Autodesk Inventor part; units mm, degrees
ref_plane "Work Plane1" through (144.7964, 60.3681, 0) normal (0.9790451, 0.2036437, 0) x (-0.2036437, 0.9790451, 0)
ref_plane "YZ Plane" through (0, 0, 0) normal (1, 0, 0) x (0, 1, 0)
ref_plane "XZ Plane" through (0, 0, 0) normal (0, 1, 0) x (-1, 0, 0)
sketch "Main Outline" plane through (0, 0, 0) normal (0, 0, 1) x (1, 0, 0)
  line L0 (0, 0) -> (304.8, 0) construction
  line L1 (304.8, 0) -> (304.8, 50.8) construction
  line L2 (304.8, 50.8) -> (0, 50.8) construction
  line L3 (0, 50.8) -> (0, 0) construction
  line L4 (0, 50.8) -> (0, 53.34) construction
  line L5 (0, 53.34) -> (304.8, 53.34) construction
  line L6 (304.8, 53.34) -> (304.8, 50.8) construction
  circle A0 centre (152.4, 23.8125) radius 17.4625 construction
  line L7 (152.4, 23.8125) -> (152.4, 0) construction
  circle A1 centre (152.4, 23.8125) radius 27.94 construction
  circle A2 centre (152.4, 23.8125) radius 21.59 construction
  line L8 (152.4, 23.8125) -> (144.7964, 60.3681) construction
  circle A3 centre (144.7964, 60.3681) radius 15.24 construction
  circle A4 centre (144.7964, 60.3681) radius 8.89 construction
  circle A5 centre (144.7964, 60.3681) radius 14.2875 construction
  arc A6 (164.6591, 71.8014) -> (129.0153, 43.7486) centre (144.7964, 60.3681) ccw construction
  circle A7 centre (98.8106, 85.598) radius 32.258 construction
  circle A8 centre (126.6733, 147.4971) radius 32.258 construction
  circle A9 centre (176.9075, 101.8424) radius 32.258 construction
  circle A10 centre (144.7964, 60.3681) radius 11.1125 construction
  circle A11 centre (152.4, 23.8125) radius 49.53 construction
  line L9 (144.7964, 60.3681) -> (126.6733, 147.4971) construction
  line L10 (144.7964, 60.3681) -> (98.8106, 85.598) construction
  line L11 (98.8106, 85.598) -> (176.9075, 101.8424) construction
  line L12 (176.9075, 101.8424) -> (144.7964, 60.3681) construction
  circle A12 centre (98.8106, 85.598) radius 9.5493 construction
  arc A13 (174.9629, 111.1915) -> (185.6989, 98.1139) centre (176.9075, 101.8424) ccw construction
  circle A14 centre (126.6733, 147.4971) radius 9.5493 construction
  line L13 (96.8659, 94.9472) -> (174.9629, 111.1915) construction
  line L14 (185.6989, 98.1139) -> (165.8956, 51.4198) construction
  line L15 (92.2351, 78.6732) -> (129.0153, 43.7486) construction
  line L16 (174.9629, 111.1915) -> (176.9075, 101.8424) construction
  line L17 (176.9075, 101.8424) -> (185.6989, 98.1139) construction
  arc A15 (185.6989, 98.1139) -> (174.9629, 111.1915) centre (176.9075, 101.8424) ccw construction
  arc A16 (165.8956, 51.4198) -> (164.6591, 71.8014) centre (144.7964, 60.3681) ccw construction
  arc A17 (129.0153, 43.7486) -> (165.8956, 51.4198) centre (144.7964, 60.3681) ccw construction
  circle A18 centre (126.6086, 147.808) radius 32.258 construction
  circle A19 centre (126.544, 148.1188) radius 32.258 construction
  circle A20 centre (126.4793, 148.4297) radius 32.258 construction
  line L18 (126.6733, 147.4971) -> (126.4793, 148.4297) construction
  circle A21 centre (126.738, 147.1863) radius 32.258 construction
  circle A22 centre (117.4622, 43.2997) radius 9.525 construction
  circle A23 centre (176.6694, 55.615) radius 9.525 construction
  line L19 (152.4, 23.8125) -> (117.4622, 43.2997) construction
  line L20 (152.4, 23.8125) -> (176.6694, 55.615) construction
  line L21 (117.4622, 43.2997) -> (98.8106, 85.598) construction
  line L22 (176.6694, 55.615) -> (176.9075, 101.8424) construction
  circle A24 centre (135.1821, 106.5897) radius 7.9375 construction
  line L23 (135.6243, 150.8242) -> (166.2787, 68.353) construction
  circle A25 centre (152.4, 23.8125) radius 29.845 construction
  line L24 (117.1381, 146.979) -> (121.9118, 59.1246) construction
  circle A26 centre (99.0889, 85.4453) radius 32.258 construction
  circle A27 centre (97.9755, 86.0562) radius 32.258 construction
  line L25 (97.9755, 86.0562) -> (98.8106, 85.598) construction
  circle A28 centre (98.2538, 85.9034) radius 32.258 construction
  circle A29 centre (98.5322, 85.7507) radius 32.258 construction
  circle A30 centre (152.4, 23.8125) radius 29.845 construction
  circle A31 centre (122.555, 23.8125) radius 6.35 construction
  circle A32 centre (179.7696, 35.7133) radius 6.35 construction
  line L26 (122.555, 23.8125) -> (152.4, 23.8125) construction
  line L27 (152.4, 23.8125) -> (182.245, 23.8125) construction
  circle A33 centre (182.245, 23.8125) radius 6.35 construction
  circle A34 centre (125.0304, 11.9117) radius 6.35 construction
  circle A35 centre (150.4199, 33.3321) radius 39.5684 construction
  line L28 (72.9795, 65.6655) -> (119.7593, 8.3204) construction
  circle A36 centre (177.4906, 102.5955) radius 32.258 construction
  line L29 (176.9075, 101.8424) -> (177.4906, 102.5955) construction
  circle A37 centre (177.2963, 102.3445) radius 32.258 construction
  circle A38 centre (177.1019, 102.0934) radius 32.258 construction
  circle A39 centre (176.7131, 101.5913) radius 32.258 construction
  line L30 (188.5109, 22.6209) -> (208.5442, 93.8632) construction
  circle A40 centre (135.1821, 106.5897) radius 9.5727 construction
  arc A41 (86.8202, 116.3239) -> (96.3065, 136.4856) centre (81.3304, 131.2195) ccw construction
  arc A42 (158.9123, 149.5077) -> (175.6513, 134.801) centre (174.7462, 150.6502) ccw construction
  line L31 (126.4793, 148.4297) -> (126.9966, 145.9429) construction
  line L32 (116.5322, 146.3607) -> (117.0495, 143.8739) construction
  line L33 (136.9437, 148.0119) -> (136.4264, 150.4987) construction
  arc A43 (136.4264, 150.4987) -> (116.5322, 146.3607) centre (126.4793, 148.4297) ccw construction
  arc A44 (117.0495, 143.8739) -> (136.9437, 148.0119) centre (126.9966, 145.9429) ccw construction
  line L34 (177.4906, 102.5955) -> (175.9357, 100.5871) construction
  line L35 (169.4571, 108.8154) -> (167.9021, 106.807) construction
  line L36 (183.9692, 94.3672) -> (185.5242, 96.3756) construction
  arc A45 (185.5242, 96.3756) -> (169.4571, 108.8154) centre (177.4906, 102.5955) ccw construction
  arc A46 (167.9021, 106.807) -> (183.9692, 94.3672) centre (175.9357, 100.5871) ccw construction
  line L37 (97.9755, 86.0562) -> (100.2023, 84.8344) construction
  line L38 (93.0884, 77.1487) -> (95.3153, 75.927) construction
  line L39 (105.0894, 93.7418) -> (102.8625, 94.9636) construction
  arc A47 (102.8625, 94.9636) -> (93.0884, 77.1487) centre (97.9755, 86.0562) ccw construction
  arc A48 (95.3153, 75.927) -> (105.0894, 93.7418) centre (100.2023, 84.8344) ccw construction
  circle A49 centre (117.4622, 43.2997) radius 3.9687 construction
  circle A50 centre (176.6694, 55.615) radius 3.9687 construction
  line L40 (152.4, 23.8125) -> (158.4777, -5.4071) construction
  arc A51 (80.1751, 59.3139) -> (79.0947, 58.1692) centre (79.7097, 58.6709) ccw construction
  arc A52 (205.9254, 84.5503) -> (204.4781, 85.1692) centre (205.1613, 84.7652) ccw construction
  circle A53 centre (152.4, 23.8125) radius 14.224 construction
  circle A54 centre (135.1821, 106.5897) radius 3.9687 construction
  circle A55 centre (156.538, 3.9183) radius 6.35 construction
  circle A56 centre (156.538, 3.9183) radius 2.0828 construction
  circle A57 centre (152.4, 23.8125) radius 20.32 construction
  line L41 (133.1021, 30.1759) -> (152.4, 23.8125) construction
  line L42 (152.4, 23.8125) -> (167.5599, 37.3432) construction
  circle A58 centre (167.5599, 37.3432) radius 2.0828 construction
  circle A59 centre (167.5599, 37.3432) radius 3.9687 construction
  circle A60 centre (133.1021, 30.1759) radius 2.0828 construction
  circle A61 centre (133.1021, 30.1759) radius 3.9688 construction
  point P0 (126.738, 147.1863)
  point P1 (176.7131, 101.5913)
  dimension "d18" = 99.06
  dimension "d58" = 64.516
  dimension "d86" = 64.516
  dimension "d0" = 304.8
  dimension "d1" = 50.8
  dimension "d2" = 2.54
  dimension "d3" = 34.925
  dimension "d4" = 23.8125
  dimension "d5" = 152.4
  dimension "d6" = 55.88
  dimension "d7" = 43.18
  dimension "d8" = 37.338
  dimension "d10" = 30.48
  dimension "d11" = 17.78
  dimension "d12" = 28.575
  dimension "d13" = 45.8366
  dimension "d14" = 64.516
  dimension "d15" = 64.516
  dimension "d16" = 64.516
  dimension "d17" = 22.225
  dimension "d19" = 52.4523
  dimension "d20" = 88.9939
  dimension "d21" = 19.0986
  dimension "d22" = 19.0986
  dimension "d23" = 19.0986
  dimension "d30" = 124.732
  dimension "d40" = 64.516
  dimension "d41" = 64.516
  dimension "d42" = 64.516
  dimension "d43" = 0.9525
  dimension "d44" = 0.3175
  dimension "d45" = 0.635
  dimension "d46" = 64.516
  dimension "d47" = 0.3175
  dimension "d48" = 19.05
  dimension "d49" = 19.05
  dimension "d50" = 40.005
  dimension "d51" = 40.005
  dimension "d52" = 46.228
  dimension "d54" = 46.228
  dimension "d55" = 15.875
  dimension "d56" = 41.4655
  dimension "d57" = 59.69
  dimension "d59" = 64.516
  dimension "d60" = 64.516
  dimension "d61" = 64.516
  dimension "d62" = 0.3175
  dimension "d63" = 0.3175
  dimension "d64" = 0.635
  dimension "d65" = 0.9525
  dimension "d73" = 12.7
  dimension "d74" = 12.7
  dimension "d76" = 59.69
  dimension "d78" = 12.7
  dimension "d79" = 12.7
  dimension "d80" = 64.516
  dimension "d81" = 0.9525
  dimension "d82" = 64.516
  dimension "d83" = 64.516
  dimension "d84" = 0.3175
  dimension "d85" = 0.635
  dimension "d88" = 0.3175
  dimension "d89" = 31.75
  dimension "d90" = 31.75
  dimension "d94" = 1.5875
  dimension "d95" = 20.32
  dimension "d96" = 1.5875
sketch "Upper CIM C-C Check" plane through (0, 0, 0) normal (0, 0, 1) x (1, 0, 0)
  arc A0 (3.4429, -22.6582) -> (3.4429, 22.6582) centre (0, 0) ccw construction
  arc A1 (90.4285, 9.4409) -> (90.4285, -9.4409) centre (88.9939, 0) ccw construction
  line L0 (88.9939, 0) -> (0, 0) construction
  line L1 (90.4285, 9.4409) -> (3.4429, 22.6582)
  line L2 (3.4429, -22.6582) -> (90.4285, -9.4409)
  arc A2 (90.4285, -9.4409) -> (90.4285, 9.4409) centre (88.9939, 0) ccw
  arc A3 (3.4429, 22.6582) -> (3.4429, -22.6582) centre (0, 0) ccw
  dimension "d24" = 45.8366
  dimension "d25" = 19.0986
  dimension "d26" = 78.9119
  dimension "d27" = 87.984
  dimension "d28" = 27.12
  dimension "d29" = 88.9939
sketch "Sketch3" plane through (0, 0, 0) normal (0, 0, 1) x (1, 0, 0)
  arc A0 (80.1751, 59.3139) -> (79.0947, 58.1692) centre (79.7097, 58.6709) ccw construction
  line L0 (72.9795, 65.6655) -> (119.7593, 8.3204) construction
  circle A1 centre (150.4199, 33.3321) radius 39.5684 construction
  line L1 (188.5109, 22.6209) -> (208.5442, 93.8632) construction
  arc A2 (205.9254, 84.5503) -> (204.4781, 85.1692) centre (205.1613, 84.7652) ccw construction
  line L2 (79.0947, 58.1692) -> (119.7593, 8.3204)
  line L3 (188.5109, 22.6209) -> (205.9254, 84.5503)
  arc A3 (119.7593, 8.3204) -> (188.5109, 22.6209) centre (150.4199, 33.3321) ccw
  line L4 (78.4796, 57.6675) -> (119.1442, 7.8187)
  arc A4 (119.1442, 7.8187) -> (189.275, 22.4061) centre (150.4199, 33.3321) ccw
  line L5 (189.275, 22.4061) -> (206.6896, 84.3354)
  line L6 (79.0947, 58.1692) -> (78.4796, 57.6675)
  line L7 (206.6896, 84.3354) -> (205.9254, 84.5503)
  point P0 (0, 0)
  dimension "d115" = 0.7937
extrude "Extrusion1" add sketch "Sketch3" along normal blind 45.2437
ref_plane "Work Plane1" through (144.7964, 60.3681, 0) normal (0.9790451, 0.2036437, 0) x (-0.2036437, 0.9790451, 0)
sketch "Sketch4" plane through (188.5109, 22.6209, 0) normal (-0.9626636, 0.2707007, 0) x (0, 0, 1)
  line L0 (0, 0) -> (0, 64.3313)
  line L1 (0, 0) -> (45.2437, 0)
  line L2 (45.2437, 64.3313) -> (45.2437, 0)
  line L3 (0, 64.3313) -> (45.2437, 64.3313)
  line L4 (3.175, 64.3313) -> (3.175, 0)
  line L5 (42.0688, 64.3313) -> (42.0688, 0)
  point P0 (0, -72.8064)
  point P1 (3.175, 45.2813)
  point P2 (42.0688, 45.2813)
  dimension "d119" = 3.175
  dimension "d120" = 3.175
  dimension "d121" = 19.05
  dimension "d122" = 19.05
hole "Hole1" at (200.7686, 66.2116, 3.175) at (200.7686, 66.2116, 42.0688) direction (0.9626636, -0.2707007, 0) diameter 2.9464 end through all
mirror "Mirror1" about plane through (144.7964, 60.3681, 0) normal (0.9790451, 0.2036437, 0) of "Hole1"
sketch "Sketch6" plane through (0, 0, 45.2437) normal (0, 0, 1) x (1, 0, 0)
  line L0 (119.7593, 8.3204) -> (79.0947, 58.1692)
  line L1 (79.0947, 58.1692) -> (78.4796, 57.6675)
  line L2 (78.4796, 57.6675) -> (119.1442, 7.8187)
  arc A0 (119.1442, 7.8187) -> (189.275, 22.4061) centre (150.4199, 33.3321) ccw
  line L3 (189.275, 22.4061) -> (206.6896, 84.3354)
  line L4 (206.6896, 84.3354) -> (205.9254, 84.5503)
  line L5 (205.9254, 84.5503) -> (188.5109, 22.6209)
  arc A1 (119.7593, 8.3204) -> (188.5109, 22.6209) centre (150.4199, 33.3321) ccw
  line L6 (46.0816, -65.5817) -> (259.8786, -42.4203)
  point P0 (0, 0)
  dimension "d135" = 86.3855
  dimension "d136" = 64.3312
  dimension "d137" = 215.048
equation "\"d3\" = r10"
equation "\"d6\" = g44"
equation "\"d7\" = g34"
equation "\"d10\" = g24"
equation "\"d11\" = g14"
equation "\"d12\" = r8"
equation "\"d13\" = p48"
equation "\"d14\" = cim"
equation "\"d15\" = cim"
equation "\"d16\" = cim"
equation "\"d17\" = r6"
equation "\"d21\" = p20"
equation "\"d22\" = p20"
equation "\"d23\" = p20"
equation "\"d24\" = p48"
equation "\"d25\" = p20"
equation "\"d29\" = d20"
equation "\"g14\" = 17.78"
equation "\"g24\" = 30.48"
equation "\"g34\" = 43.18"
equation "\"g44\" = 55.88"
equation "\"p20\" = 19.09859"
equation "\"p48\" = 45.83662"
equation "\"r10\" = 34.925"
equation "\"r9\" = 31.75"
equation "\"r8\" = 28.575"
equation "\"r7\" = 25.4"
equation "\"r6\" = 22.225"
equation "\"r5\" = 19.05"
equation "\"r4\" = 15.875"
equation "\"r3\" = 12.7"
equation "\"cim\" = 64.516"
equation "\"act\" = 28.448"
equation "\"actL\" = 23.749"
equation "\"UpperCimCCCheck\" = 2 * d27 + d26 + d28"
equation "\"LowerBeltPathCCCheck\" = 267"
equation "\"SheildArc\" = 215.04798"
properties material "Aluminum 6061"
Source: CAD feature listing. Evaluate the final solid. Frame: model axes, mm. A direction names the side the tool comes from. Coordinates: 2 decimals unless noted, no trailing zeros. Order: outer loops, then holes, each group sorted by start corner. A loop starts at its lowest first (then second) coordinate and runs counter-clockwise, first axis right, second up.
Item 1: Cut plane B-B (z = 6). Return loops of the section in (x, y) (1 decimal), plus the area to 3 significant figures.
Output values:
outline: (78.5, 57.7) - (119.1, 7.8) arc R40.4 ccw to (189.3, 22.4) - (206.7, 84.3) - (205.9, 84.6) - (188.5, 22.6) arc R39.6 cw to (119.8, 8.3) - (79.1, 58.2) - close
area: 171 mm2
Item 2: Set-up query: faces 3 (the face through (98.53, 33.09, 22.31)), 4 (the face through (99.142, 33.594, 22.305)). Return all of +Z, -Z, +X, -X, +Y, -Y with unobstructed straight access to the full face (end or side cutting, diameter ignored); none if empty.
Output values:
face 3: +Z, -Z, -X, -Y
face 4: +Z, -Z, +Y
Item 3: Pull-direction query (Z, two-part tool) for faces 1 (the face through (201.036, 65.677, 43.474)), 2 (the face through (197.096, 53.152, 22.305)); classes: pulls with the +Z half, pulls with the -Z half, needs draft (parallel to the pull), parting line crosses it, or undercut.
Output values:
face 1: undercut
face 2: needs draft
Item 4: Cut plane A-A (y = 34). Return loops of the section in (x, z), plus the area to 3 significant figures.
Output values:
outline: (97.79, 0) - (98.81, 0) - (98.81, 45.24) - (97.79, 45.24) - close; (191.71, 0) - (192.54, 0) - (192.54, 45.24) - (191.71, 45.24) - close
area: 83.7 mm2
Item 5: Cut plane D-D (x = 191). Return loops of the section in (y, z), plus the area to 3 significant figures.
Output values:
outline: (28.54, 0) - (31.47, 0) - (31.47, 45.24) - (28.54, 45.24) - close
area: 133 mm2
Item 6: Cut plane C-C (y = 1.5). Return loops of the section in (x, z).
Output values:
outline: (125.6, 0) - (126.92, 0) - (126.92, 45.24) - (125.6, 45.24) - close; (173.92, 0) - (175.24, 0) - (175.24, 45.24) - (173.92, 45.24) - close
Item 7: First-contact query: P1, Ø12, axis at x = 110, y = 36.5, coming from the -Z side; P2, Ø10, axis at x = 142.5, z = 29, coming from the +Y side; P3, Ø1, axis at x = 165.5, z = 40, coming from the -Y side; P4, Ø1, axis at x = 139, z = 17.5, coming from the -Y side. Flat tips, straight axial feed; report the tip coordinate or a pass-through.
Output values:
P1: passes through
P2: stops at y = -4.07
P3: stops at y = -4.3
P4: stops at y = -5.52
Item 8: Material intervals for line 1 (Y direction, x = 150, z = 22.5); line 2 (X direction, y = 5.5, z = 4); line 3 (X direction, y = 13, z = 24), sorted ascending.
Output values:
line 1: y = -7.03 to -6.23
line 2: x = 121.19 to 122.29, 178.55 to 179.65
line 3: x = 114.92 to 115.94, 184.36 to 185.29
